Autodesk Inventor part; units mm, degrees
ref_plane "YZ Plane" through (0, 0, 0) normal (1, 0, 0) x (0, 1, 0)
ref_plane "XZ Plane" through (0, 0, 0) normal (0, 1, 0) x (-1, 0, 0)
ref_plane "XY Plane" through (0, 0, 0) normal (0, 0, 1) x (1, 0, 0)
sketch "Sketch1" plane through (0, 0, 0) normal (0, 0, 1) x (1, 0, 0)
  line L0 (-12.9018, 8.1017) -> (137.0982, 8.1017)
  line L1 (137.0982, 8.1017) -> (137.0982, -141.8983)
  line L2 (137.0982, -141.8983) -> (-12.9018, -141.8983)
  line L3 (-12.9018, -141.8983) -> (-12.9018, 8.1017)
  point P0 (0, 0)
  dimension "d0" = 150
  dimension "d1" = 150
extrude "Extrusion1" add sketch "Sketch1" along normal blind 150
sketch "Sketch2" plane through (-12.9018, 8.1017, 0) normal (0, 1, 0) x (1, 0, 0)
  point P0 (12.9018, 0)
ref_plane "Work Plane1" through (-12.9018, 1.7517, 0) normal (0, 1, 0) x (1, 0, 0)
sketch "Sketch3" plane through (-12.9018, 1.7517, 0) normal (0, 1, 0) x (1, 0, 0)
  line L0 (6.35, -143.65) -> (143.65, -143.65)
  line L1 (143.65, -143.65) -> (143.65, -6.35)
  line L2 (143.65, -6.35) -> (6.35, -6.35)
  line L3 (6.35, -6.35) -> (6.35, -143.65)
  line L4 (150, -150) -> (0, -150)
  line L5 (0, 0) -> (0, -150)
  point P0 (12.9018, 0)
  dimension "d5" = 137.3
  dimension "d6" = 137.3
  dimension "d7" = 6.35
  dimension "d8" = 6.35
loft "Loft1" cut profiles "Sketch3" section 1 edges at (62.0982, 8.1017, 0) (-12.9018, 8.1017, 75) (62.0982, 8.1017, 150) (137.0982, 8.1017, 75)
sketch "Sketch4" plane through (-6.5518, 1.7517, 6.35) normal (0, 1, 0) x (1, 0, 0)
  line L0 (0, -137.3) -> (137.3, -137.3)
  line L1 (137.3, -137.3) -> (137.3, 0)
  line L2 (0, -137.3) -> (137.3, -137.3)
  line L3 (137.3, -137.3) -> (137.3, 0)
  line L4 (137.3, 0) -> (0, 0)
  line L5 (0, 0) -> (0, -137.3)
  point P0 (6.5518, 6.35)
extrude "Extrusion2" cut sketch "Sketch4" against normal blind 137.3
properties part number "insulationbox"
Here's how the part is built. I have some questions about the finished solid (model axes, mm). A direction names the side the tool comes from. Round coordinates to 2 decimals unless told otherwise and drop trailing zeros. Loops run counter-clockwise (first coordinate to the right, second up) from the corner with the lowest first, then second, coordinate; pieces in that order, holes last.
1. If I drill on line 1 along Z through (x, y) = (3, -71); line 2 along X through (y, z) = (-49.5, 35); line 3 along Y through (x, z) = (41, 100), over which ranges is the centre line in solid material (lowest first)?
Answer list:
line 1: z = 0 to 6.35, 143.65 to 150
line 2: x = -12.9 to -6.55, 130.75 to 137.1
line 3: y = -141.9 to -135.55
2. We'd pull the mould along X, two halves only. Please class faces 1 (the face through (-12.902, -68, 74)), 2 (the face through (63, -141.898, 74)), 3 (the face through (63, -66, 6.35)): +X half, -X half, draft (parallel to the pull), parting line (faces both ways), or undercut.
Answer list:
face 1: -X half
face 2: draft
face 3: undercut
3. Which directions (+Z, -Z, +X, -X, +Y, -Y) give clear straight access to the entire face, cutting with the end or side of a thin tool? Please do faces 4 (the face through (61, -66, 143.65)), 5 (the face through (61, -66, 0)).
Answer list:
face 4: +Y
face 5: -Z, +X, -X, +Y, -Y
4. If we section it at A-A on y = -10: Write out the boundary of the cut face in (x, z), plus the area to 3 significant figures.
Answer list:
outline: (-12.9, 0) - (137.1, 0) - (137.1, 150) - (-12.9, 150) - close; hole (-6.55, 6.35) - (130.75, 6.35) - (130.75, 143.65) - (-6.55, 143.65) - close
area: 3,650 mm2
5. For P1, Ø8, axis at x = 24.5, y = -67.5, coming from the -Z side; P2, Ø5, axis at x = 79.5, z = 53.5, coming from the +Y side, each with a flat end and sliding along its axis, tell me the tip position at first contact or that it passes through.
Answer list:
P1: stops at z = 0
P2: stops at y = -135.55
